from build123d import *

# Parameters (mm, degrees)
SKETCH1_W               = 396.24
SKETCH1_H               = 19.05
CUT_EXTRUDE1_DEPTH      = 101.6
CUT_EXTRUDE1_DEPTH_BACK = 69.088
BOSS_EXTRUDE1_START     = 125.15372202
BOSS_EXTRUDE1_OUTLINE_R = 25.273
BOSS_EXTRUDE1_DEPTH     = 260.35


# Read off the part's stored shape, not the designer's step: Boss-Extrude1
with BuildPart() as part:
    # Sketch1 → Revolve1 (revolve)
    with BuildSketch(Plane.XY, mode=Mode.PRIVATE) as revolve1_sk:
        with Locations((178.556917264, 9.525)):
            Rectangle(SKETCH1_W, SKETCH1_H)
    revolve(revolve1_sk.sketch.rotate(Axis((-62.064477949, 19.05, 0), (1, 0, 0)), 270), axis=Axis((-62.064477949, 19.05, 0), (1, 0, 0)))

    # 3DSketch1 → Cut-Extrude1 (cut, two sides: drawn at the far end of the back side and taken through both)
    with BuildSketch(Plane(origin=(125.15372202, 38.1, 0), x_dir=(-0.9587579392690639, -0.2842238798703196, 0), z_dir=(0, 0, -1)).offset(-CUT_EXTRUDE1_DEPTH_BACK)):
        Polygon((0, 0), (12.838737839, -43.308260512), (158.928287458, 0), (141.370884548, 59.225493089), (-6.410822017, 15.415592494), align=None)
    extrude(amount=CUT_EXTRUDE1_DEPTH + CUT_EXTRUDE1_DEPTH_BACK, mode=Mode.SUBTRACT)

    # Boss-Extrude1 outline → Boss-Extrude1 (add)
    with BuildSketch(Plane.YZ.offset(BOSS_EXTRUDE1_START)):
        with Locations((19.05, 0)):
            Circle(BOSS_EXTRUDE1_OUTLINE_R)
    extrude(amount=BOSS_EXTRUDE1_DEPTH)


solid = part.part
Read the model definition and answer for the solid it produces. Units are mm, in the model's axes. Coordinates: 2 decimals unless noted, no trailing zeros. Loops run counter-clockwise (first coordinate to the right, second up) from the corner with the lowest first, then second, coordinate; pieces in that order, holes last. Notation, with made-up numbers: (-4.5, 65) -> (9.5, 65) arc R22 ccw to (9.5, 76) -> close; hole circle Ø2 at (43, 57). An arc over 180 degrees is marked (long way). Write item = value, one per line. Start each with the question number.
1) The part is cut by section D-D, the plane y = 34.5. Determine the outline of the cut face in (x, z).
2) The part is cut by section A-A, the plane x = 348. Determine the outline of the cut face in (y, z), plus the area to 3 significant figures.
3) Find the intervals of material crossed by L1, parallel to Z at x = 182, y = 17.5; L2, parallel to Z at x = 299, y = 18; L3, parallel to Y at x = 187.5, z = -0.5, in increasing order. Write a range as from..to.
4) The part is cut by section B-B, the plane z = -12.5. Determine the outline of the cut face in (x, y).
5) Given P1, Ø6, axis at x = 155.5, z = -6.5, coming from the -Y side; P2, Ø8, axis at x = 212.5, z = 10, coming from the +Y side; P3, Ø5, axis at x = 237, z = 14, coming from the -Y side (3 decimals), each flat-ended and moving along its own axis, determine where each tip first touches the part or whether it passes through.
6) The part is cut by section C-C, the plane y = 3. Determine the outline of the cut face in (x, z), plus the area to 3 significant figures.
Result:
q1.outline = (125.15, -20) -> (385.5, -20) -> (385.5, 20) -> (125.15, 20) -> close
q2.outline = circle Ø50.55 at (19.05, 0)
q2.area = 2,010 mm²
q3.L1 = -25.23..25.23
q3.L2 = -25.25..25.25
q3.L3 = -6.22..44.32
q4.outline = (125.15, -2.92) -> (385.5, -2.92) -> (385.5, 41.02) -> (125.15, 41.02) -> close
q5.P1 = -5.98
q5.P2 = 43.6
q5.P3 = -3.455
q6.outline = (125.15, -19.52) -> (385.5, -19.52) -> (385.5, 19.52) -> (125.15, 19.52) -> close
q6.area = 10,200 mm²
